Design review of the part built by this model. Coordinates are the model's own, in mm. A direction names the side the tool comes from. Coordinates: 2 decimals unless noted, no trailing zeros. Write each loop counter-clockwise with the first axis right and the second up, starting at its lowest first coordinate (ties: lowest second). Pieces come first, ordered by that corner, then holes. Notation, with made-up numbers: (57, 56.25) - (106, 56.25) arc R18 cw to (106, 79.25) - close; hole circle Ø8 at (-20, 49.25). An arc over 180 degrees is marked (long way). One line per item, written item: value.
from build123d import *

# Parameters (mm, degrees)
SKETCH_1_R          = 14
SKETCH_1_R_2        = 1.5
EXTRUDE_1_DEPTH     = 5
SKETCH_2_R          = 13
SKETCH_2_R_2        = 4.5
CUT_EXTRUDE_1_DEPTH = 2
SKETCH_3_R          = 1.5
CUT_EXTRUDE_2_DEPTH = 21.420577857
SKETCH_4_R          = 4
CUT_EXTRUDE_3_DEPTH = 3
CUT_EXTRUDE_4_DEPTH = 4
FILLET_1_R          = 2
EXTRUDE_START       = 14
SKETCH_6_R          = 11
SKETCH_6_R_2        = 1.5
EXTRUDE_3_DEPTH     = 14
FILLET_2_R          = 2


with BuildPart() as part:
    # 草图1 → 凸台-拉伸1 (new body)
    with BuildSketch(Plane(origin=(0, 0, 0), x_dir=(1, 0, 0), z_dir=(0, 1, 0))):
        with Locations(Location((0, 0, 0), (0, 0, 270))):
            Circle(SKETCH_1_R)
        with Locations(Location((-9.5, 0, 0), (0, 0, 270))):
            Circle(SKETCH_1_R_2, mode=Mode.SUBTRACT)
        with Locations(Location((9.5, 0, 0), (0, 0, 270))):
            Circle(SKETCH_1_R_2, mode=Mode.SUBTRACT)
        with Locations(Location((0, 8, 0), (0, 0, 270))):
            Circle(SKETCH_1_R_2, mode=Mode.SUBTRACT)
        with Locations(Location((0, -8, 0), (0, 0, 270))):
            Circle(SKETCH_1_R_2, mode=Mode.SUBTRACT)
    extrude(amount=EXTRUDE_1_DEPTH)

    # 草图2 → 切除-拉伸1 (cut)
    with BuildSketch(Plane(origin=(0, 5, 0), x_dir=(1, 0, 0), z_dir=(0, 1, 0))):
        with Locations(Location((0, 0, 0), (0, 0, 270))):
            Circle(SKETCH_2_R)
        with Locations(Location((0, 0, 0), (0, 0, 270))):
            Circle(SKETCH_2_R_2, mode=Mode.SUBTRACT)
    extrude(amount=-CUT_EXTRUDE_1_DEPTH, mode=Mode.SUBTRACT)

    # 草图3 → 切除-拉伸2 (cut, through all)
    with BuildSketch(Plane(origin=(0, 5, 0), x_dir=(1, 0, 0), z_dir=(0, 1, 0))):
        with Locations(Location((0, 0, 0), (0, 0, 270))):
            Circle(SKETCH_3_R)
    extrude(amount=-CUT_EXTRUDE_2_DEPTH, mode=Mode.SUBTRACT)

    # 草图4 → 切除-拉伸3 (cut)
    with BuildSketch(Plane.XZ):
        with Locations(Location((0, 0, 0), (0, 0, 270))):
            Circle(SKETCH_4_R)
    extrude(amount=-CUT_EXTRUDE_3_DEPTH, mode=Mode.SUBTRACT)

    # 草图5 → 切除-拉伸4 (cut)
    with BuildSketch(Plane.XZ):
        with BuildLine():
            Line((8.485281374, 4.242640687), (11.790860146, 7.548219459))
            ThreePointArc((11.790860146, 7.548219459), (9.899494937, 9.899494937), (7.548219459, 11.790860146))
            Line((7.548219459, 11.790860146), (4.242640687, 8.485281374))
            ThreePointArc((4.242640687, 8.485281374), (4.242640687, 4.242640687), (8.485281374, 4.242640687))
        make_face()
        with BuildLine():
            Line((8.485281374, -4.242640687), (11.790860146, -7.548219459))
            ThreePointArc((11.790860146, -7.548219459), (9.899494937, -9.899494937), (7.548219459, -11.790860146))
            Line((7.548219459, -11.790860146), (4.242640687, -8.485281374))
            ThreePointArc((4.242640687, -8.485281374), (4.242640687, -4.242640687), (8.485281374, -4.242640687))
        make_face()
        with BuildLine():
            Line((-4.242640687, -8.485281374), (-7.548219459, -11.790860146))
            ThreePointArc((-7.548219459, -11.790860146), (-9.899494937, -9.899494937), (-11.790860146, -7.548219459))
            Line((-11.790860146, -7.548219459), (-8.485281374, -4.242640687))
            ThreePointArc((-8.485281374, -4.242640687), (-4.242640687, -4.242640687), (-4.242640687, -8.485281374))
        make_face()
        with BuildLine():
            Line((-8.485281374, 4.242640687), (-11.790860146, 7.548219459))
            ThreePointArc((-11.790860146, 7.548219459), (-9.899494937, 9.899494937), (-7.548219459, 11.790860146))
            Line((-7.548219459, 11.790860146), (-4.242640687, 8.485281374))
            ThreePointArc((-4.242640687, 8.485281374), (-4.242640687, 4.242640687), (-8.485281374, 4.242640687))
        make_face()
    extrude(amount=-CUT_EXTRUDE_4_DEPTH, mode=Mode.SUBTRACT)

    # 圆角1
    fillet_1_edges = [part.edges().sort_by_distance(p)[0] for p in [
        (3.932426601, 0, 13.436369339),
        (14, 0, 0),
        (0, 0, -14),
        (-14, 0, 0),
    ]]
    fillet(fillet_1_edges, radius=FILLET_1_R)

    # 草图6 → 凸台-拉伸3 (add)
    with BuildSketch(Plane(origin=(0, 5, 0), x_dir=(1, 0, 0), z_dir=(0, 1, 0)).offset(EXTRUDE_START)):
        with Locations(Location((0, 0, 0), (0, 0, 270))):
            Circle(SKETCH_6_R)
        with Locations(Location((0, 0, 0), (0, 0, 270))):
            Circle(SKETCH_6_R_2, mode=Mode.SUBTRACT)
    extrude(amount=-EXTRUDE_3_DEPTH)

    # 圆角2
    fillet_2_edges = [part.edges().sort_by_distance(p)[0] for p in [
        (0, 19, -11),
    ]]
    fillet(fillet_2_edges, radius=FILLET_2_R)


solid = part.part
1. Consider section A-A, the plane x = 0. Give the number of separate pieces and of enclosed holes in the cut face, then the cut area to 3 significant figures.
Answer block:
separate pieces: 4
enclosed holes: 0
area: 321 mm^2
2. Mouldability with a two-part tool opening along Y and no side actions: class faces 1 (the face through (-5, 0, 0)), 2 (the face through (-5.87, 1.53, -10.11)), 3 (the face through (0, 3, 6)) as released by +Y, released by -Y, zero draft, split by the parting line, or undercut.
Answer block:
face 1: released by -Y
face 2: zero draft
face 3: undercut
3. Consider section B-B, the plane y = 13.5. Write out the cut boundary in (x, z).
Answer block:
outline: circle Ø22 at (0, 0); hole circle Ø3 at (0, 0)
4. Insertion check: pin 1 Ø4 at (x, z) = (-8.5, 9) entering from -Y; pin 2 Ø5 at (y, z) = (5.5, 8.5) entering from -X (3 decimals); pin 3 Ø1.5 at (x, z) = (6, -5.5) entering from -Y. Each pin has a flat end and moves straight along its axis. Give the tip position at first contact, or say it passes through.
Answer block:
pin 1: stops at y = 4
pin 2: stops at x = -12.625
pin 3: stops at y = 5
5. For faces 4 (the face through (1.352, 4.014, 4.292)), 5 (the face through (10.11, 1.53, -5.87)), 6 (the face through (5.92, 1.53, -10.16)), list the 3-axis set-ups (+Z, -Z, +X, -X, +Y, -Y) from which the entire face can be reached by the end or side of a thin tool; tool diameter is ignored.
Answer block:
face 4: none
face 5: -Z, -Y
face 6: +X, -Y
6. Wall thickness on line 1 along Y through (x, z) = (-0.25, 5.25); line 2 along X through (y, z) = (2.25, 6.75); line 3 along Y through (x, z) = (1, 11.5): over which ranges is each line inside the solid? List them lowest first.
Answer block:
line 1: y = 0 to 3, 5 to 19
line 2: x = -12.27 to -10.99, -3.39 to -0.83, 0.83 to 3.39, 10.99 to 12.27
line 3: y = 0 to 3
